Autodesk Fusion 360 part; units mm, degrees
sketch "Sketch1" plane through (0, 0, 0) normal (0, 0, 1) x (1, 0, 0)
  line L0 (-7.5, 0) -> (7.5, 0)
  line L1 (7.5, 0) -> (7.5, 275)
  line L2 (7.5, 275) -> (-7.5, 275)
  line L3 (-7.5, 275) -> (-7.5, 0)
  line L4 (-7.5, 7) -> (-4.5, 7)
  line L5 (-4.5, 7) -> (-4.5, 11)
  line L6 (-4.5, 11) -> (-7.5, 11)
  line L7 (0, 0) -> (0, 275)
  dimension "d1" = 15
  dimension "d2" = 275
  dimension "d3" = 7
  dimension "d4" = 4
  dimension "d5" = 3
revolve "Revolve1" add sketch "Sketch1" angle 360 about axis through (0, 0, 0) along (0, 1, 0) contours L0 L1 L2 L7
extrude "Extrude1" cut sketch "Sketch1" along normal through all and the other way through all contours L3 L4 L5 L6
mirror "Mirror1" about plane through (0, 0, 0) normal (1, 0, 0) of "Extrude1"
ref_plane "WorkPlane1" through (0, 137.5, 0) normal (0, -1, 0) x (0, 0, -1)
hole "Hole2" at (0, 0, 0) direction (0, 1, 0) diameter 1.5 depth 5 tip angle 118
mirror "Mirror2" about plane through (0, 137.5, 0) normal (0, -1, 0) of "Mirror1", "Extrude1", "Hole2"
chamfer "Chamfer1" distance 0.5 angle 45 2 edges at (-6.9925, 0, -2.7121) (-6.9925, 275, -2.7121)
Read the model definition and answer for the solid it produces. Units are mm, in the model's axes. Round coordinates to 2 decimals unless told otherwise and drop trailing zeros. Order: outer loops, then holes, each group sorted by start corner. A loop starts at its lowest first (then second) coordinate and runs counter-clockwise, first axis right, second up.
1) The part is cut by section A-A on y = 50.5. Write down the section's boundary in (x, z), plus the area to 3 significant figures.
2) Straight lines are drawn through the part: L1, parallel to Y at x = -5, z = -4; L2, parallel to X at y = 3.7, z = 0. For each, find the intervals that lie inside material, in ascending order.
3) Flat-ended cylindrical pins translate along their axes: pin 1 (2 mm diameter, centred on y = 9, z = 1.5, fed in from -X); pin 2 (3 mm diameter, centred on x = 3, y = 197.5, fed in from -Z); pin 3 (3 mm diameter, centred on y = 267, z = -2.5, fed in from -X). Find the tip coordinate at first contact, or state that the pin passes through.
Resolved:
1. outline: circle Ø15 at (0, 0)
1. area: 177 mm2
2. L1: y = 0 to 7, 11 to 264, 268 to 275
2. L2: x = -7.5 to -0.75, 0.75 to 7.5
3. pin 1: stops at x = -4.5
3. pin 2: stops at z = -7.35
3. pin 3: stops at x = -7.37
